CAD build for the part. Positions are in the model's coordinates, mm. Coordinates: 2 decimals unless noted, no trailing zeros. Loops run counter-clockwise (first coordinate to the right, second up) from the corner with the lowest first, then second, coordinate; pieces in that order, holes last. Notation, with made-up numbers: (-15.5, 81) -> (-3.5, 81) arc R10 ccw to (-3.5, 98) -> close; hole circle Ø9 at (88.5, 57). An arc over 180 degrees is marked (long way). Write each question's results on one line, items separated by ' | '.
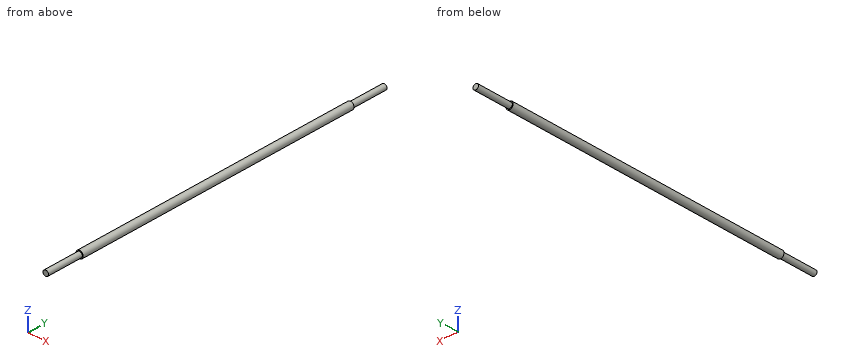
```python
from build123d import *

# Parameters (mm, degrees)
F0_R      = 10
F1_DEPTH  = 500
F1_FACE_R = 10
F2_DEPTH  = 500
F3_R      = 10
F3_R_2    = 7.5
F4_DEPTH  = 100
F5_R      = 10
F5_R_2    = 7.5
F6_DEPTH  = 100


with BuildPart() as f1:
    # F0 (on Front) → F1 (new body)
    with BuildSketch(Plane.XZ):
        Circle(F0_R)
    extrude(amount=F1_DEPTH)

    # F1_face (on face) → F2 (join)
    with BuildSketch(Plane(origin=(0, 0, 0), x_dir=(1, 0, 0), z_dir=(0, 1, 0))):
        Circle(F1_FACE_R)
    extrude(amount=F2_DEPTH)

    # F3 (on face) → F4 (cut)
    with BuildSketch(Plane(origin=(0, 500, 0), x_dir=(-1, 0, 0), z_dir=(0, 1, 0))):
        Circle(F3_R)
        Circle(F3_R_2, mode=Mode.SUBTRACT)
    extrude(amount=-F4_DEPTH, mode=Mode.SUBTRACT)

    # F5 (on face) → F6 (cut)
    with BuildSketch(Plane.XZ.offset(500)):
        Circle(F5_R)
        Circle(F5_R_2, mode=Mode.SUBTRACT)
    extrude(amount=-F6_DEPTH, mode=Mode.SUBTRACT)


solid = f1.part
```
Q1. Cut at C-C on y = -164. Write the cut outline in (x, z), and give its area (3 significant figures).
Results are:
outline: circle Ø20 at (0, 0) | area: 314 mm^2
Q2. Cut at A-A on z = 0. Write the cut outline in (x, y), and give its area (3 significant figures).
Results are:
outline: (-10, -400) -> (-7.5, -400) -> (-7.5, -500) -> (7.5, -500) -> (7.5, -400) -> (10, -400) -> (10, 400) -> (7.5, 400) -> (7.5, 500) -> (-7.5, 500) -> (-7.5, 400) -> (-10, 400) -> close | area: 19,000 mm^2
Q3. Cut at B-B on x = 0. Write the cut outline in (y, z), and give its area (3 significant figures).
Results are:
outline: (-500, -7.5) -> (-400, -7.5) -> (-400, -10) -> (400, -10) -> (400, -7.5) -> (500, -7.5) -> (500, 7.5) -> (400, 7.5) -> (400, 10) -> (-400, 10) -> (-400, 7.5) -> (-500, 7.5) -> close | area: 19,000 mm^2
Q4. Drop flat-ended pins along their axis: pin 1 (8 mm diameter, centred on y = 235, z = 7, fed in from +X); pin 2 (5 mm diameter, centred on x = -8, y = 6, fed in from +Z). Give the stop position or say it passes through.
Results are:
pin 1: x = 9.54 | pin 2: z = 8.35
Q5. Wall check: L1, parallel to Y at x = -3, z = -8.5; L2, parallel to X at y = 206.5, z = -1.75; L3, parallel to Z at x = 6.75, y = -238. Give the ranges that are in metal, low to high. Write a range as from..to.
Results are:
L1: -400..400 | L2: -9.85..9.85 | L3: -7.38..7.38
